The listing builds one solid part. Answer for the finished solid, in the listing's coordinates (mm). A direction names the side the tool comes from. Give positions to 0.01 mm unless a question says otherwise; leave off trailing zeros. Loops run counter-clockwise (first coordinate to the right, second up) from the corner with the lowest first, then second, coordinate; pieces in that order, holes last. Notation, with made-up numbers: (17, 40) - (23, 40) arc R21 ccw to (23, 71) - close; hole circle Ø4 at (30, 37.25). An arc over 180 degrees is marked (long way). Answer in a Markdown table with one row per item. Add a question column.
Autodesk Fusion 360 part; units mm, degrees
sketch "side" plane through (0, 0, 0) normal (0, 1, 0) x (1, 0, 0)
  line L0 (0, 0) -> (55, 0)
  line L1 (55, 0) -> (55, -25)
  line L2 (55, -25) -> (70, -50)
  line L3 (70, -50) -> (0, -50)
  line L4 (0, -50) -> (0, 0)
  dimension "d1" = 70
  dimension "d2" = 59.036
  dimension "d3" = 50
  dimension "d4" = 25
extrude "Extrude1" add sketch "side" along normal blind 240
shell "Shell1" thickness 5 removed faces 1 at (46.6667, 80, 50)
sketch "actuator hole" plane through (0, 0, 0) normal (0, -1, 0) x (1, 0, 0)
  line L0 (70, 50) -> (0, 50)
  line L1 (0, 50) -> (0, 0)
  line L2 (0, 0) -> (55, 0)
  line L3 (55, 0) -> (55, 25)
  line L4 (55, 25) -> (70, 50)
  circle A0 centre (35, 25) radius 5
  line L5 (35, 50) -> (35, 0)
  line L6 (0, 25) -> (15, 25)
  line L7 (15, 25) -> (55, 25)
  dimension "d8" = 10
extrude "Extrude2" cut sketch "actuator hole" against normal blind 230 contours A0 L5 L7 | A0 L5 L7 | A0 L5 L7 | A0 L5 L7
(1) A cutting plane is placed at B-B on x = 35. Determine the outline of the cut face in (y, z), plus the area to 3 significant figures.
(2) A cutting plane is placed at A-A on z = 14.5. Determine the outline of the cut face in (x, y), plus the area to 3 significant figures.
(3) A tool of negligible diameter and unlimited length cuts with its end or side. For faces 4 (the face through (27, 118, 5)), 5 (the face through (31, 2, 22)), 6 (the face through (55, 118, 12)), from which of +Z, -Z, +X, -X, +Y, -Y can it reach the whole face along a straight path? Write none if from no direction.
(4) A cutting plane is placed at D-D on x = 59.5. Determine the outline of the cut face in (y, z).
(5) Given pin 1 Ø20 at (y, z) = (148.5, 8.5) entering from +X; pin 2 Ø6 at (x, y) = (54, 155.5) entering from +Z; pin 3 Ø1 at (x, y) = (22.5, 175) entering from +Z, each flat-ended and moving along its own axis, determine where each tip first touches the part or whether it passes through.
(6) Find the intervals of material crossed by line 1 along X through (y, z) = (1.6, 25); line 2 along Y through (x, z) = (53, 44); line 3 along X through (y, z) = (25, 17.5), in increasing order. Write a range as [from, to].
(7) A cutting plane is placed at C-C on y = 152.5. Determine the outline of the cut face in (x, z).
(8) The mould has two halves that part along X. Classify faces 1 (the face through (50, 118, 16)), 2 (the face through (66, 102, 50)), 3 (the face through (62.395, 118.32, 37.325)): pulls with the +X half, pulls with the -X half, needs draft (parallel to the pull), parting line crosses it, or undercut.
Evaluation:
| question | item | result |
|---|---|---|
| 1 | outline | (0, 0) - (240, 0) - (240, 50) - (235, 50) - (235, 5) - (5, 5) - (5, 20) - (0, 20) - close; (0, 30) - (5, 30) - (5, 50) - (0, 50) - close |
| 1 | area | 1,600 mm² |
| 2 | outline | (0, 0) - (55, 0) - (55, 240) - (0, 240) - close; hole (5, 5) - (50, 5) - (50, 235) - (5, 235) - close |
| 2 | area | 2,850 mm² |
| 3 | face 4 | +Z |
| 3 | face 5 | -Y |
| 3 | face 6 | -Z, +X, +Y, -Y |
| 4 | outline | (0, 32.5) - (240, 32.5) - (240, 50) - (235, 50) - (235, 42.22) - (5, 42.22) - (5, 50) - (0, 50) - close |
| 5 | pin 1 | stops at x = 55 |
| 5 | pin 2 | stops at z = 38.05 |
| 5 | pin 3 | stops at z = 5 |
| 6 | line 1 | x = [0, 30], [40, 55] |
| 6 | line 2 | y = [0, 5], [235, 240] |
| 6 | line 3 | x = [0, 5], [50, 55] |
| 7 | outline | (0, 0) - (55, 0) - (55, 25) - (70, 50) - (64.17, 50) - (50, 26.38) - (50, 5) - (5, 5) - (5, 50) - (0, 50) - close |
| 8 | face 1 | undercut |
| 8 | face 2 | needs draft |
| 8 | face 3 | pulls with the +X half |
